Source: CAD feature listing. Evaluate the final solid. Frame: model axes, mm. Face numbers are marked on the shaded views. A direction names the side the tool comes from. Coordinates: 2 decimals unless noted, no trailing zeros. Write each loop counter-clockwise with the first axis right and the second up, starting at its lowest first coordinate (ties: lowest second). Pieces come first, ordered by that corner, then holes. Notation, with made-up numbers: M 69,-30 L 117,-30 A10 ccw 117,-13 Z; hole C 16,55.25 d11. An arc over 180 degrees is marked long. Answer as CSV lines item,"result". Start each with the question number.
1. Line query: probe 1 along Y at (x, z) = (2, 8.75); probe 2 along Z at (x, y) = (0, 3.5); probe 3 along X at (y, z) = (45, 7.5). Output: solid intervals per line, ascending. Write a range as [from, to].
2. Contact query for flat-ended pins moving along their axis: pin 1 Ø6 at (y, z) = (25, 4.5) entering from +X; pin 2 Ø2 at (y, z) = (-25.5, 3) entering from +X; pin 3 Ø2 at (x, y) = (7, -9) entering from +Z. Output: stop coordinate, or through.
3. Section D-D on z = -8. Return the cut outline in (x, y), plus the area to 3 significant figures.
4. Section A-A on z = 0. Return the cut outline in (x, y).
5. Section C-C on y = 18. Return the cut outline in (x, z), plus the area to 3 significant figures.
6. Section B-B on x = 0. Return the cut outline in (y, z).
7. Reachability of the marked faces 1, 2 and 3 from +Z, -Z, +X, -X, +Y, -Y: full face, straight path, thin tool, end or side. Return the list, or none.
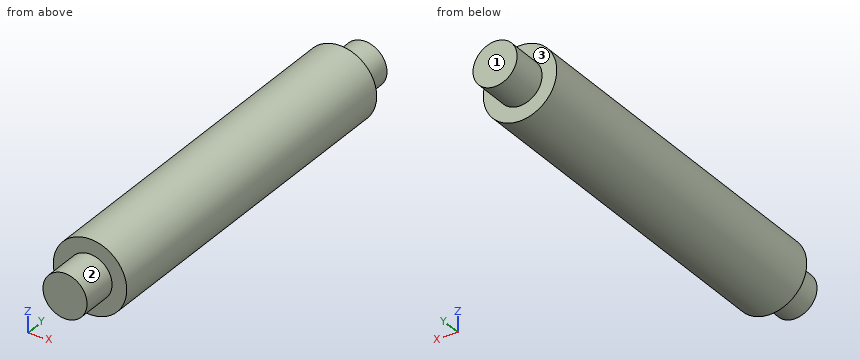
Autodesk Inventor part; units mm, degrees
ref_plane "YZ Plane" through (0, 0, 0) normal (1, 0, 0) x (0, 1, 0)
ref_plane "XZ Plane" through (0, 0, 0) normal (0, 1, 0) x (-1, 0, 0)
ref_plane "XY Plane" through (0, 0, 0) normal (0, 0, 1) x (1, 0, 0)
sketch "草圖1" plane through (0, 0, 0) normal (0, 0, 1) x (1, 0, 0)
  line L0 (0, 50) -> (10, 50)
  line L1 (10, 50) -> (10, -50)
  line L2 (10, -50) -> (0, -50)
  line L3 (0, -50) -> (0, 50)
  line L4 (0, 50) -> (6, 50)
  line L5 (6, 50) -> (6, 60)
  line L6 (6, 60) -> (0, 60)
  line L7 (0, 60) -> (0, 50)
  line L8 (0, -50) -> (6, -50)
  line L9 (6, -50) -> (6, -60)
  line L10 (6, -60) -> (0, -60)
  line L11 (0, -60) -> (0, -50)
  point P0 (0, 0)
  point P1 (10, 0)
  dimension "d0" = 10
  dimension "d1" = 6
  dimension "d2" = 6
  dimension "d3" = 120
  dimension "d4" = 100
  dimension "d5" = 10
revolve "迴轉1" add sketch "草圖1" angle 360 about axis through (0, -50, 0) along (0, 1, 0)
properties part number "P9"
Values:
1,probe 1,"[-50, 50]"
1,probe 2,"[-10, 10]"
1,probe 3,"[-6.61, 6.61]"
2,pin 1,"x = 9.89"
2,pin 2,"x = 9.8"
2,pin 3,"z = 8"
3,outline,"M -6,-50 L 6,-50 L 6,50 L -6,50 Z"
3,area,"1,200 mm²"
4,outline,"M -10,-50 L -6,-50 L -6,-60 L 6,-60 L 6,-50 L 10,-50 L 10,50 L 6,50 L 6,60 L -6,60 L -6,50 L -10,50 Z"
5,outline,"C 0,0 d20"
5,area,"314 mm²"
6,outline,"M -60,-6 L -50,-6 L -50,-10 L 50,-10 L 50,-6 L 60,-6 L 60,6 L 50,6 L 50,10 L -50,10 L -50,6 L -60,6 Z"
7,face 1,"+Z, -Z, +X, -X, +Y"
7,face 2,"-Y"
7,face 3,"+Y"
